Source: CAD feature listing. Evaluate the final solid. Frame: model axes, mm. Face numbers are marked on the shaded views. A direction names the side the tool comes from. Give positions to 0.01 mm unless a question says otherwise; leave off trailing zeros. Loops run counter-clockwise (first coordinate to the right, second up) from the corner with the lowest first, then second, coordinate; pieces in that order, holes last. Notation, with made-up numbers: M 63.5,74.5 L 72.5,74.5 A20 cw 72.5,81.5 Z; hole C 22,-15.75 d7. An arc over 180 degrees is marked long. Answer in a Markdown table with one row per item.
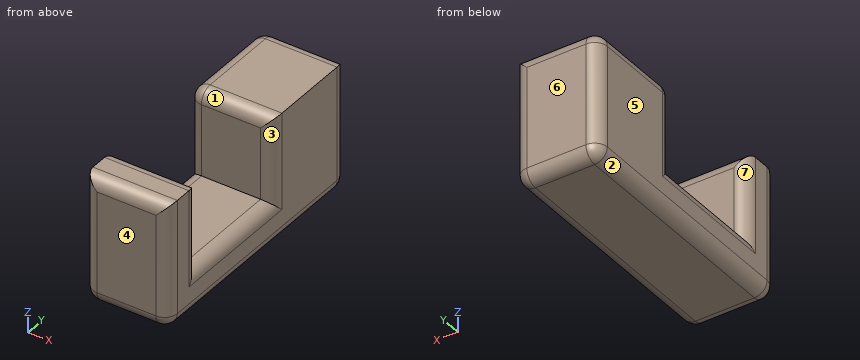
```python
from build123d import *

# Parameters (mm, degrees)
F1_DEPTH = 20
F2_R     = 3


with BuildPart() as f1:
    # F0 (on Right) → F1 (new body)
    with BuildSketch(Plane.YZ):
        Polygon((0, 30), (0, 0), (61, 0), (61, 30), (36, 30), (36, 10), (10, 10), (10, 30), align=None)
    extrude(amount=F1_DEPTH)

    # F2
    f2_edges = [f1.edges().sort_by_distance(p)[0] for p in [
        (20, 30.5, 0),
        (10, 0, 0),
        (20, 0, 15),
        (0, 0, 15),
        (0, 30.5, 0),
        (10, 0, 30),
        (10, 61, 0),
        (0, 61, 15),
        (20, 61, 15),
        (10, 61, 30),
        (20, 23, 10),
        (20, 36, 20),
        (20, 10, 20),
        (10, 10, 30),
        (10, 36, 30),
        (0, 48.5, 30),
        (0, 23, 10),
        (0, 36, 20),
        (0, 10, 20),
    ]]
    fillet(f2_edges, radius=F2_R)


solid = f1.part
```
Q1. Ray query, probe 1 along Y at (x, z) = (6, 24); probe 2 along Z at (x, y) = (16.5, 20); probe 3 along Y at (x, z) = (2, 26). Return the intervals inside material, ascending. Write a range as from..to.
Values follow:
| item | result |
|---|---|
| probe 1 | 0..10, 36..61 |
| probe 2 | 0..10 |
| probe 3 | 0.17..9.83, 36.17..60.83 |
Q2. Section query C-C (x = 8). Output: boundary loops of the cut face in (y, z), plus the area to 3 significant figures.
Values follow:
| item | result |
|---|---|
| outline | M 0,3 A3 ccw 3,0 L 58,0 A3 ccw 61,3 L 61,27 A3 ccw 58,30 L 39,30 A3 ccw 36,27 L 36,10 L 10,10 L 10,27 A3 ccw 7,30 L 3,30 A3 ccw 0,27 Z |
| area | 1,300 mm^2 |
Q3. Section query D-D (x = 18.5). Output: boundary loops of the cut face in (y, z).
Values follow:
| item | result |
|---|---|
| outline | M 0.4,3 A2.6 ccw 3,0.4 L 58,0.4 A2.6 ccw 60.6,3 L 60.6,28.5 A3 ccw 58,30 L 39,30 A3 ccw 36.4,28.5 L 36.4,9.6 L 9.6,9.6 L 9.6,28.5 A3 ccw 7,30 L 3,30 A3 ccw 0.4,28.5 Z |
Q4. Reachability of the marked faces 1, 2 and 3 from +Z, -Z, +X, -X, +Y, -Y: full face, straight path, thin tool, end or side. Return the list, or none.
Values follow:
| item | result |
|---|---|
| face 1 | +Z, +X, -X |
| face 2 | -Z, -X, +Y, -Y |
| face 3 | +Z, +X |
Q5. Section query A-A (z = 17). Output: boundary loops of the cut face in (x, y), plus the area to 3 significant figures.
Values follow:
| item | result |
|---|---|
| outline | M 0,3 A3 ccw 3,0 L 17,0 A3 ccw 20,3 L 20,7 A3 ccw 17,10 L 3,10 A3 ccw 0,7 Z; M 0,39 A3 ccw 3,36 L 17,36 A3 ccw 20,39 L 20,58 A3 ccw 17,61 L 3,61 A3 ccw 0,58 Z |
| area | 685 mm^2 |
Q6. Mould query, pull axis Y, two halves, no side actions, for the marked faces 4, 5, 6 and 7. Classes: +Y half, -Y half, draft (parallel to the pull), parting line (faces both ways), or undercut.
Values follow:
| item | result |
|---|---|
| face 4 | -Y half |
| face 5 | draft |
| face 6 | +Y half |
| face 7 | undercut |
Q7. Section query B-B (y = 19.5). Output: boundary loops of the cut face in (x, z), plus the area to 3 significant figures.
Values follow:
| item | result |
|---|---|
| outline | M 0,3 A3 ccw 3,0 L 17,0 A3 ccw 20,3 L 20,7 A3 ccw 17,10 L 3,10 A3 ccw 0,7 Z |
| area | 192 mm^2 |
